```python
from build123d import *

# Parameters (mm, degrees)
HGR_HGR20_1_DEPTH                                   = 350
CBORE_FOR_M5_HEX_SOCKET_HEAD_CAP_SCREW1_D           = 5.8
CBORE_FOR_M5_HEX_SOCKET_HEAD_CAP_SCREW1_CBORE_D     = 10
CBORE_FOR_M5_HEX_SOCKET_HEAD_CAP_SCREW1_CBORE_DEPTH = 8.5
LPATTERN1_COUNT                                     = 6
LPATTERN1_PITCH                                     = 60.7


with BuildPart() as part:
    # Sketch12 → Hgr HGR20(1) (new body)
    with BuildSketch(Plane.XY):
        with BuildLine():
            Line((-9, 0), (9, 0))
            Line((9, 0), (10, 1))
            Line((10, 1), (10, 3.656507036))
            ThreePointArc((10, 3.656507036), (9.92387953, 4.039190479), (9.707106773, 4.363613837))
            Line((9.707106773, 4.363613837), (6.892893227, 7.177827383))
            ThreePointArc((6.892893227, 7.177827383), (6.67612047, 7.502250741), (6.6, 7.884934184))
            Line((6.6, 7.884934184), (6.6, 9.445065806))
            ThreePointArc((6.6, 9.445065806), (6.67612047, 9.827749249), (6.892893227, 10.152172607))
            Line((6.892893227, 10.152172607), (7.63016236, 10.88944174))
            ThreePointArc((7.63016236, 10.88944174), (7.773916168, 11.035785916), (7.84680643, 11.2275378))
            ThreePointArc((7.84680643, 11.2275378), (8.396388337, 12.262927707), (9.431778248, 12.812509604))
            ThreePointArc((9.431778248, 12.812509604), (9.57149389, 12.861817745), (9.690625667, 12.949905047))
            Line((9.690625667, 12.949905047), (9.85355341, 13.11283279))
            ThreePointArc((9.85355341, 13.11283279), (9.961939771, 13.275044443), (10, 13.466386134))
            Line((10, 13.466386134), (10, 14.523613846))
            ThreePointArc((10, 14.523613846), (9.961939771, 14.714955537), (9.85355341, 14.87716719))
            Line((9.85355341, 14.87716719), (9.678500884, 15.052219716))
            ThreePointArc((9.678500884, 15.052219716), (9.560417671, 15.13974885), (9.421985128, 15.189159636))
            ThreePointArc((9.421985128, 15.189159636), (8.395921997, 15.736919373), (7.84816225, 16.7629825))
            ThreePointArc((7.84816225, 16.7629825), (7.7751915, 16.95300083), (7.63253117, 17.09818942))
            Line((7.63253117, 17.09818942), (7.23072061, 17.49999998))
            Line((7.23072061, 17.49999998), (-7.23072061, 17.49999998))
            Line((-7.23072061, 17.49999998), (-7.63253117, 17.09818942))
            ThreePointArc((-7.63253117, 17.09818942), (-7.775191493, 16.953000826), (-7.84816225, 16.7629825))
            ThreePointArc((-7.84816225, 16.7629825), (-8.395921988, 15.736919382), (-9.421985103, 15.189159641))
            ThreePointArc((-9.421985103, 15.189159641), (-9.560417671, 15.139748844), (-9.678500907, 15.052219693))
            Line((-9.678500907, 15.052219693), (-9.85355341, 14.87716719))
            ThreePointArc((-9.85355341, 14.87716719), (-9.961939771, 14.714955537), (-10, 14.523613846))
            Line((-10, 14.523613846), (-10, 13.466386134))
            ThreePointArc((-10, 13.466386134), (-9.961939771, 13.275044443), (-9.85355341, 13.11283279))
            Line((-9.85355341, 13.11283279), (-9.690625709, 12.949905089))
            ThreePointArc((-9.690625709, 12.949905089), (-9.571493891, 12.861817755), (-9.431778202, 12.812509595))
            ThreePointArc((-9.431778202, 12.812509595), (-8.39638832, 12.26292769), (-7.84680643, 11.2275378))
            ThreePointArc((-7.84680643, 11.2275378), (-7.773916172, 11.035785914), (-7.63016236, 10.88944174))
            Line((-7.63016236, 10.88944174), (-6.892893227, 10.152172607))
            ThreePointArc((-6.892893227, 10.152172607), (-6.67612047, 9.827749249), (-6.6, 9.445065806))
            Line((-6.6, 9.445065806), (-6.6, 7.884934184))
            ThreePointArc((-6.6, 7.884934184), (-6.67612047, 7.502250741), (-6.892893227, 7.177827383))
            Line((-6.892893227, 7.177827383), (-9.707106773, 4.363613837))
            ThreePointArc((-9.707106773, 4.363613837), (-9.92387953, 4.039190479), (-10, 3.656507036))
            Line((-10, 3.656507036), (-10, 1))
            Line((-10, 1), (-9, 0))
        make_face()
    extrude(amount=HGR_HGR20_1_DEPTH)

    # CBORE for M5 Hex Socket Head Cap Screw1 (through all)
    with Locations(Plane(origin=(0, 17.49999998, 0), x_dir=(1, 0, 0), z_dir=(0, 1, 0))):
        with Locations((0, -25)):
            cbore_for_m5_hex_socket_head_cap_screw1 = CounterBoreHole(CBORE_FOR_M5_HEX_SOCKET_HEAD_CAP_SCREW1_D / 2, CBORE_FOR_M5_HEX_SOCKET_HEAD_CAP_SCREW1_CBORE_D / 2, CBORE_FOR_M5_HEX_SOCKET_HEAD_CAP_SCREW1_CBORE_DEPTH)

    # LPattern1: CBORE for M5 Hex Socket Head Cap Screw1 ×6
    with Locations(*[(0, 0, i * LPATTERN1_PITCH) for i in range(1, LPATTERN1_COUNT)]):
        add(cbore_for_m5_hex_socket_head_cap_screw1, mode=Mode.SUBTRACT)


solid = part.part
```
Geometry check sheet. Reference: the model listing, model coordinates, mm. A direction names the side the tool comes from. Round coordinates to 2 decimals unless told otherwise and drop trailing zeros. Return JSON: item names as keys, results as strings. Group by question number.
Q1. Section check A-A, the plane x = 0. Count the separate pieces of the cut face and the enclosed holes in it, plus the area to 3 significant figures.
Q2. Gauge pin test, flat ends, axial feed: pin 1 (3 mm diameter, centred on x = 0, z = 206.5, fed in from +Y); pin 2 (6 mm diameter, centred on x = 0, z = 267.8, fed in from +Y); pin 3 (1.5 mm diameter, centred on y = 9.5, z = 233.5, fed in from -X); pin 4 (1.5 mm diameter, centred on y = 4.5, z = 209, fed in from -X). Record the tip position at first contact, or that the pin passes through.
Q3. Tool access check on faces 4 (the flat face through (2.2, 9, 209.3)), 5 (the cylindrical face through (0.63, 4.44, 149.23)). Record the directions out of +Z, -Z, +X, -X, +Y, -Y that give a thin tool (end or side, any length) a straight path to the whole face; none if there is none.
Q4. Material ranges on probe 1 along X at (y, z) = (2, 146.4); probe 2 along X at (y, z) = (11.25, 146.4); probe 3 along Y at (x, z) = (-8.25, 331), recorded low to high. Write a range as from..to.
Q5. Release check for a two-part mould opening along Z. For faces 1 (the flat face through (0, 0, 173)), 2 (the flat face through (2.2, 9, 27.2)), 3 (the flat face through (0, 9, 350)) record: released by +Z, released by -Z, zero draft, split by the parting line, or undercut.
Numbers:
{
 "1": {"separate pieces": "7", "enclosed holes": "0", "area": "5,300 mm^2"},
 "2": {"pin 1": "through", "pin 2": "y = 9", "pin 3": "x = -6.99", "pin 4": "x = -10"},
 "3": {"face 4": "+Y", "face 5": "+Y, -Y"},
 "4": {"probe 1": "-10..-2.9, 2.9..10", "probe 2": "-7.85..-5, 5..7.85", "probe 3": "0..5.82, 12.1..15.9"},
 "5": {"face 1": "zero draft", "face 2": "undercut", "face 3": "released by +Z"}
}
